```python
from build123d import *

# Parameters (mm, degrees)
SKETCH1_W           = 57.21
SKETCH1_H           = 50
BOSS_EXTRUDE1_DEPTH = 34.8
SKETCH2_R           = 2.5
CUT_EXTRUDE1_DEPTH  = 51


with BuildPart() as part:
    # Sketch1 → Boss-Extrude1 (new body)
    with BuildSketch(Plane(origin=(0, 0, 0), x_dir=(1, 0, 0), z_dir=(0, 1, 0))):
        Rectangle(SKETCH1_W, SKETCH1_H)
    extrude(amount=BOSS_EXTRUDE1_DEPTH)

    # Sketch2 → Cut-Extrude1 (cut, through all)
    with BuildSketch(Plane.XY.offset(25)):
        with Locations((-12.72, 13.45)):
            Circle(SKETCH2_R)
    cut_extrude1 = extrude(amount=-CUT_EXTRUDE1_DEPTH, mode=Mode.SUBTRACT)

    # Mirror1: Cut-Extrude1 across plane
    add(cut_extrude1.mirror(Plane(origin=(0, 0, 0), x_dir=(0, 0, 1), z_dir=(1, 0, 0))), mode=Mode.SUBTRACT)


solid = part.part
```
For this review, take the finished solid that the model builds, in its own axes (mm). Coordinates: 2 decimals unless noted, no trailing zeros. Order: outer loops, then holes, each group sorted by start corner. A loop starts at its lowest first (then second) coordinate and runs counter-clockwise, first axis right, second up. Notation, with made-up numbers: (73.5, -35.5) -> (120.5, -35.5) arc R20 ccw to (120.5, 0.5) -> close; hole circle Ø6 at (35, 19.5). An arc over 180 degrees is marked (long way). Use CSV: the item, a comma, the result in double quotes. Start each with the question number.
Item 1: Insertion check: pin 1 (8 mm diameter, centred on x = -12.72, y = 13.45, fed in from -Z). The pin has a flat end and moves straight along its axis. Give the tip position at first contact, or say it passes through.
Item 2: We need section B-B, the plane x = -12.72. Give the boundary of the cut face in (y, z), then the cut area to 3 significant figures.
Item 3: We need section A-A, the plane y = 13.45. Give the boundary of the cut face in (x, z) (3 decimals), then the cut area to 3 significant figures.
Item 4: Wall thickness on probe 1 along X at (y, z) = (13, 3) (3 decimals); probe 2 along Y at (x, z) = (-12.72, 15.5); probe 3 along Y at (x, z) = (-12, -17): over which ranges is each line inside the solid? List them lowest first.
Item 5: We need section C-C, the plane z = 3. Give the boundary of the cut face in (x, y) (3 decimals).
Item 6: Draft analysis for pull direction Y (two halves, no side actions). For faces 1 (the face through (-10.41, 12.49, 0.35)), 2 (the face through (28.605, 17, 0)), 3 (the face through (0, 34.8, 0)), state which applies: pulls with the +Y half, pulls with the -Y half, needs draft (parallel to the pull), parting line crosses it, or undercut.
Derived:
1,pin 1,"stops at z = -25"
2,outline,"(0, -25) -> (10.95, -25) -> (10.95, 25) -> (0, 25) -> close; (15.95, -25) -> (34.8, -25) -> (34.8, 25) -> (15.95, 25) -> close"
2,area,"1,490 mm^2"
3,outline,"(-28.605, -25) -> (-15.22, -25) -> (-15.22, 25) -> (-28.605, 25) -> close; (-10.22, -25) -> (10.22, -25) -> (10.22, 25) -> (-10.22, 25) -> close; (15.22, -25) -> (28.605, -25) -> (28.605, 25) -> (15.22, 25) -> close"
3,area,"2,360 mm^2"
4,probe 1,"x = -28.605 to -15.179, -10.261 to 10.261, 15.179 to 28.605"
4,probe 2,"y = 0 to 10.95, 15.95 to 34.8"
4,probe 3,"y = 0 to 11.06, 15.84 to 34.8"
5,outline,"(-28.605, 0) -> (28.605, 0) -> (28.605, 34.8) -> (-28.605, 34.8) -> close; hole circle Ø5 at (-12.72, 13.45); hole circle Ø5 at (12.72, 13.45)"
6,face 1,"undercut"
6,face 2,"needs draft"
6,face 3,"pulls with the +Y half"
